The model under review builds one solid part; all positions refer to its coordinate system, in mm. Face numbers are marked on the shaded views. A direction names the side the tool comes from. Coordinates: 2 decimals unless noted, no trailing zeros. Order: outer loops, then holes, each group sorted by start corner. A loop starts at its lowest first (then second) coordinate and runs counter-clockwise, first axis right, second up.
```python
from build123d import *

# Parameters (mm, degrees)
F1_R            = 11.1125
F1_R_2          = 8.3058
F2_DEPTH        = 12.7
F4_DEPTH        = 12.7
F4_COPIES_COUNT = 10


# Not quite as in the source:
# - a pattern or mirror of a feature is missing from the dataset's text; its kind, count and spacing are read off the source's solid


with BuildPart() as f2:
    # F1 (on Front) → F2 (new body)
    with BuildSketch(Plane.XZ):
        Circle(F1_R)
        Circle(F1_R_2, mode=Mode.SUBTRACT)
    extrude(amount=F2_DEPTH)

    # F3 (on face) → F4 (join, through all)
    with BuildSketch(Plane(origin=(0, 0, 0), x_dir=(-1, 0, 0), z_dir=(0, 1, 0))):
        with BuildLine():
            ThreePointArc((-2.0497311639, 8.0489077393), (-1.5602325902, 7.9743573542), (-1.2730759239, 7.5709869752))
            Line((-1.2730759239, 7.5709869752), (-1.239895929, 7.4213216903))
            ThreePointArc((-1.239895929, 7.4213216903), (0, 6.4262), (1.239895929, 7.4213216903))
            Line((1.239895929, 7.4213216903), (1.2730759239, 7.5709869752))
            ThreePointArc((1.2730759239, 7.5709869752), (1.5602325902, 7.9743573542), (2.0497311639, 8.0489077393))
            ThreePointArc((2.0497311639, 8.0489077393), (0, 8.3058), (-2.0497311639, 8.0489077393))
        make_face()
    f4 = extrude(amount=-F4_DEPTH)

    # F4_copies: F4 ×10 about axis
    f4_copies_axis = Axis((0, 0, 0), (0, 1, 0))
    for i in range(1, F4_COPIES_COUNT):
        add(f4.rotate(f4_copies_axis, i * 360 / F4_COPIES_COUNT))


solid = f2.part
```
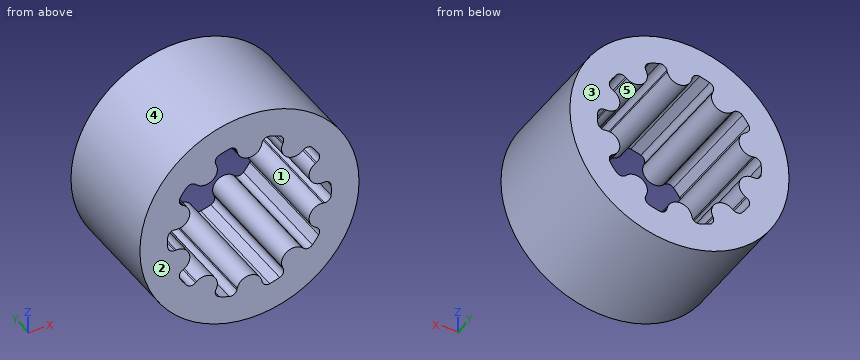
(1) Draft analysis for pull direction X (two halves, no side actions). For the marked faces 3, 4 and 5, state which applies: released by +X, released by -X, zero draft, split by the parting line, or undercut.
A:
face 3: zero draft
face 4: split by the parting line
face 5: undercut
(2) For pin 1 Ø1 at (x, y) = (-5, -3.5) entering from +Z; pin 2 Ø2 at (y, z) = (-3.5, -8) entering from +X; pin 3 Ø5 at (x, y) = (-9, -5.5) entering from +Z, all flat-tipped, find the tip position at first contact; note any pin that passes through.
A:
pin 1: stops at z = 10.16
pin 2: stops at x = 8.63
pin 3: stops at z = 9.01
(3) We need section B-B, the plane z = 0. Write out the cut boundary in (x, y), and give its area (3 significant figures).
A:
outline: (-11.11, -12.7) - (-8.31, -12.7) - (-8.31, 0) - (-11.11, 0) - close; (8.31, -12.7) - (11.11, -12.7) - (11.11, 0) - (8.31, 0) - close
area: 71.3 mm2
(4) We need section A-A, the plane x = 0. Write out the cut boundary in (y, z), and give its area (3 significant figures).
A:
outline: (-12.7, -11.11) - (0, -11.11) - (0, -6.43) - (-12.7, -6.43) - close; (-12.7, 6.43) - (0, 6.43) - (0, 11.11) - (-12.7, 11.11) - close
area: 119 mm2
(5) Machinability: for the marked faces 1 and 2, which of the approach directions +Z, -Z, +X, -X, +Y, -Y give a long, thin tool a straight path to every point of the face, cutting with its end or side? Answer none if there is none.
A:
face 1: +Y, -Y
face 2: +Z, -Z, +X, -X, -Y
(6) Wall thickness on probe 1 along Z at (x, y) = (6.75, -9.75); probe 2 along X at (y, z) = (-0.5, -7.25); probe 3 along X at (y, z) = (-12, 4): over which ranges is each line inside the solid? List them lowest first.
A:
probe 1: z = -8.83 to -4.84, -3.52 to -1.24, 1.24 to 3.52, 4.84 to 8.83
probe 2: x = -8.42 to -3.46, -1.19 to 1.19, 3.46 to 8.42
probe 3: x = -10.37 to -7.11, 7.11 to 10.37
(7) We need section C-C, the plane x = 9.25. Write out the cut boundary in (y, z), and give its area (3 significant figures).
A:
outline: (-12.7, -6.16) - (0, -6.16) - (0, 6.16) - (-12.7, 6.16) - close
area: 156 mm2
